Geometry check sheet. Reference: the model listing, model coordinates, mm. A direction names the side the tool comes from. Coordinates: 2 decimals unless noted, no trailing zeros. Write each loop counter-clockwise with the first axis right and the second up, starting at its lowest first coordinate (ties: lowest second). Pieces come first, ordered by that corner, then holes.
from build123d import *

# Parameters (mm, degrees)
SKETCH1_W              = 34.925
SKETCH1_H              = 31.75
PLATE_DEPTH            = 4
F_10_CLEARANCE_HOLE1_D = 5.1054
LOAD_CELL_CUTOUT_REACH = 26.919
FILLET1_R              = 3.175
CUT_EXTRUDE1_REACH     = 26.919
SKETCH5_R              = 2.6035
CHAMFER1_SIZE          = 0.508


with BuildPart() as part:
    # Sketch1 → Plate (new, symmetric)
    with BuildSketch(Plane(origin=(0, 0, 0), x_dir=(1, 0, 0), z_dir=(0, 1, 0))):
        Rectangle(SKETCH1_W, SKETCH1_H)
    extrude(amount=PLATE_DEPTH, both=True)

    # #10 Clearance Hole1 (through all)
    with Locations(Plane(origin=(0, 4, 0), x_dir=(1, 0, 0), z_dir=(0, 1, 0))):
        with Locations((-12.7, 11.1125), (12.7, 11.1125), (12.7, -11.1125), (-12.7, -11.1125)):
            Hole(F_10_CLEARANCE_HOLE1_D / 2)

    # Sketch4 → Load Cell Cutout (cut, up to next)
    with BuildSketch(Plane(origin=(0, 4, 0), x_dir=(1, 0, 0), z_dir=(0, 1, 0)), mode=Mode.PRIVATE) as load_cell_cutout_sk1:
        with BuildLine():
            Line((11.009869163, 6.927542495), (17.078427656, 5.008))
            Line((17.078427656, 5.008), (22.733, 5.008))
            Line((22.733, 5.008), (22.733, -5.008))
            Line((22.733, -5.008), (17.078427656, -5.008))
            Line((17.078427656, -5.008), (11.009869163, -6.927542495))
            ThreePointArc((11.009869163, -6.927542495), (-13.008, 0), (11.009869163, 6.927542495))
        make_face()
    load_cell_cutout_tool1 = extrude(load_cell_cutout_sk1.sketch, amount=-LOAD_CELL_CUTOUT_REACH, mode=Mode.PRIVATE) & part.part
    add(load_cell_cutout_tool1.solids().sort_by_distance((2.977457, 4, 0))[0], mode=Mode.SUBTRACT)

    # Fillet1
    fillet1_edges = [part.edges().sort_by_distance(p)[0] for p in [
        (11.009869163, 0, 6.927542495),
        (11.009869163, 0, -6.927542495),
    ]]
    fillet(fillet1_edges, radius=FILLET1_R)

    # Sketch5 → Cut-Extrude1 (cut, up to next)
    with BuildSketch(Plane(origin=(0, 4, 0), x_dir=(1, 0, 0), z_dir=(0, 1, 0)), mode=Mode.PRIVATE) as cut_extrude1_sk1:
        with Locations(Location((-12.7, 11.1125, 0), (0, 0, 270))):
            Circle(SKETCH5_R)
    cut_extrude1_tool1 = extrude(cut_extrude1_sk1.sketch, amount=-CUT_EXTRUDE1_REACH, mode=Mode.PRIVATE) & part.part
    # Sketch5 → Cut-Extrude1 (cut, up to next)
    with BuildSketch(Plane(origin=(0, 4, 0), x_dir=(1, 0, 0), z_dir=(0, 1, 0)), mode=Mode.PRIVATE) as cut_extrude1_sk2:
        with Locations(Location((12.7, 11.1125, 0), (0, 0, 270))):
            Circle(SKETCH5_R)
    cut_extrude1_tool2 = extrude(cut_extrude1_sk2.sketch, amount=-CUT_EXTRUDE1_REACH, mode=Mode.PRIVATE) & part.part
    # Sketch5 → Cut-Extrude1 (cut, up to next)
    with BuildSketch(Plane(origin=(0, 4, 0), x_dir=(1, 0, 0), z_dir=(0, 1, 0)), mode=Mode.PRIVATE) as cut_extrude1_sk3:
        with Locations(Location((-12.7, -11.1125, 0), (0, 0, 270))):
            Circle(SKETCH5_R)
    cut_extrude1_tool3 = extrude(cut_extrude1_sk3.sketch, amount=-CUT_EXTRUDE1_REACH, mode=Mode.PRIVATE) & part.part
    # Sketch5 → Cut-Extrude1 (cut, up to next)
    with BuildSketch(Plane(origin=(0, 4, 0), x_dir=(1, 0, 0), z_dir=(0, 1, 0)), mode=Mode.PRIVATE) as cut_extrude1_sk4:
        with Locations(Location((12.7, -11.1125, 0), (0, 0, 270))):
            Circle(SKETCH5_R)
    cut_extrude1_tool4 = extrude(cut_extrude1_sk4.sketch, amount=-CUT_EXTRUDE1_REACH, mode=Mode.PRIVATE) & part.part
    add(cut_extrude1_tool1.solids().sort_by_distance((-12.7, 4, -11.1125))[0], mode=Mode.SUBTRACT)
    add(cut_extrude1_tool2.solids().sort_by_distance((12.7, 4, -11.1125))[0], mode=Mode.SUBTRACT)
    add(cut_extrude1_tool3.solids().sort_by_distance((-12.7, 4, 11.1125))[0], mode=Mode.SUBTRACT)
    add(cut_extrude1_tool4.solids().sort_by_distance((12.7, 4, 11.1125))[0], mode=Mode.SUBTRACT)

    # Chamfer1
    # the kernel refuses this chamfer: 0.508 mm, written as the material it takes off along each edge
    with BuildSketch(Plane(origin=(13.009505309, -4, -9.625084967), x_dir=(-0.30158215810749167, 0, 0.9534401931485937), z_dir=(0.9534401931485937, 0, 0.30158215810749167))) as chamfer1_piece_1:
        Polygon((3.175 - CHAMFER1_SIZE, 0), (3.175, -CHAMFER1_SIZE), (3.175, 0), align=None)
    revolve(axis=Axis((13.009505309, -4, -9.625084967), (0, -1, 0)), revolution_arc=35.951449602, mode=Mode.SUBTRACT)
    with BuildSketch(Plane(origin=(18.324016186, -4, -4.614008558), x_dir=(0.30146813499365677, -0.02749587661058555, -0.9530797135354744), z_dir=(-0.9534401931485939, 0, -0.30158215810749184)), Plane(origin=(12.051981957, -4, 6.597912354), x_dir=(0.30146813499365605, -0.02749587661058387, 0.9530797135354745), z_dir=(0.9534401931485941, 0, -0.30158215810749117))) as chamfer1_piece_2:
        Polygon((CHAMFER1_SIZE * 0.999621916911, -CHAMFER1_SIZE * 0.0274958766106), (-CHAMFER1_SIZE * 0.0274958766106, -CHAMFER1_SIZE * 0.999621916911), (0, 0), align=None)
    extrude(amount=6.578319516, mode=Mode.SUBTRACT)
    with BuildSketch(Plane(origin=(17.4625, -4, -3.701585042), x_dir=(-0.9996219169112968, -0.027495876610585605, 0), z_dir=(0, 0, -1)), Plane(origin=(17.4625, -4, 17.181414958), x_dir=(-0.9996219169112968, -0.027495876610585605, 0), z_dir=(0, 0, -1))) as chamfer1_piece_3:
        Polygon((CHAMFER1_SIZE * 0.999621916911, CHAMFER1_SIZE * 0.0274958766106), (-CHAMFER1_SIZE * 0.0274958766106, CHAMFER1_SIZE * 0.999621916911), (0, 0), align=None)
    extrude(amount=13.479829916, mode=Mode.SUBTRACT)
    with BuildSketch(Plane(origin=(18.768914958, -4, -15.875), x_dir=(0, -0.027495876610585605, 0.9996219169112968), z_dir=(-1, 0, 0)), Plane(origin=(-18.768914958, -4, 15.875), x_dir=(0, -0.027495876610585605, -0.9996219169112968), z_dir=(1, 0, 0))) as chamfer1_piece_4:
        Polygon((CHAMFER1_SIZE * 0.999621916911, CHAMFER1_SIZE * 0.0274958766106), (-CHAMFER1_SIZE * 0.0274958766106, CHAMFER1_SIZE * 0.999621916911), (0, 0), align=None)
    extrude(amount=37.537829916, mode=Mode.SUBTRACT)
    with BuildSketch(Plane(origin=(-17.4625, -4, -17.181414958), x_dir=(0.9996219169112968, -0.027495876610585605, 0), z_dir=(0, 0, 1))) as chamfer1_piece_5:
        Polygon((CHAMFER1_SIZE * 0.999621916911, CHAMFER1_SIZE * 0.0274958766106), (-CHAMFER1_SIZE * 0.0274958766106, CHAMFER1_SIZE * 0.999621916911), (0, 0), align=None)
    extrude(amount=34.362829916, mode=Mode.SUBTRACT)
    with BuildSketch(Plane(origin=(13.009505309, -4, 9.625084967), x_dir=(-0.8038994814723275, 0, -0.5947651836553002), z_dir=(-0.5947651836553002, 0, 0.8038994814723275))) as chamfer1_piece_6:
        Polygon((3.175 - CHAMFER1_SIZE, 0), (3.175, -CHAMFER1_SIZE), (3.175, 0), align=None)
    revolve(axis=Axis((13.009505309, -4, 9.625084967), (0, -1, 0)), revolution_arc=35.951449602, mode=Mode.SUBTRACT)
    with BuildSketch(Plane(origin=(0, -4, 0), x_dir=(0.8038994814723273, 0, -0.5947651836553005), z_dir=(0.5947651836553005, 0, 0.8038994814723273))) as chamfer1_piece_7:
        Polygon((13.008 + CHAMFER1_SIZE, 0), (13.008, CHAMFER1_SIZE), (13.008, 0), align=None)
    revolve(axis=Axis((0, -4, 0), (0, 1, 0)), revolution_arc=287.00821123, mode=Mode.SUBTRACT)
    with BuildSketch(Plane(origin=(-12.7, -4, -11.1125), x_dir=(0, 0, 1), z_dir=(-1, 0, 0))) as chamfer1_piece_8:
        Polygon((2.6035 + CHAMFER1_SIZE, 0), (2.6035, CHAMFER1_SIZE), (2.6035, 0), align=None)
    revolve(axis=Axis((-12.7, -4, -11.1125), (0, 1, 0)), mode=Mode.SUBTRACT)
    with BuildSketch(Plane(origin=(12.7, -4, -11.1125), x_dir=(0, 0, 1), z_dir=(-1, 0, 0))) as chamfer1_piece_9:
        Polygon((2.6035 + CHAMFER1_SIZE, 0), (2.6035, CHAMFER1_SIZE), (2.6035, 0), align=None)
    revolve(axis=Axis((12.7, -4, -11.1125), (0, 1, 0)), mode=Mode.SUBTRACT)
    with BuildSketch(Plane(origin=(-12.7, -4, 11.1125), x_dir=(0, 0, 1), z_dir=(-1, 0, 0))) as chamfer1_piece_10:
        Polygon((2.6035 + CHAMFER1_SIZE, 0), (2.6035, CHAMFER1_SIZE), (2.6035, 0), align=None)
    revolve(axis=Axis((-12.7, -4, 11.1125), (0, 1, 0)), mode=Mode.SUBTRACT)
    with BuildSketch(Plane(origin=(12.7, -4, 11.1125), x_dir=(0, 0, 1), z_dir=(-1, 0, 0))) as chamfer1_piece_11:
        Polygon((2.6035 + CHAMFER1_SIZE, 0), (2.6035, CHAMFER1_SIZE), (2.6035, 0), align=None)
    revolve(axis=Axis((12.7, -4, 11.1125), (0, 1, 0)), mode=Mode.SUBTRACT)


solid = part.part
1. Draft check along Z on faces 1 (the cylindrical face through (-10.12, 0.31, 10.77)), 2 (the flat face through (0, 0, -15.875)), 3 (the flat face through (17.462, 0, 11)). Enter one of: released by +Z, released by -Z, zero draft, split by the parting line, or undercut.
Computed values:
face 1: undercut
face 2: released by -Z
face 3: zero draft
2. Sectioned sample at C-C, the plane z = 0. Record the boundary of the cut face in (x, y).
Computed values:
outline: (-17.46, -3.49) - (-16.95, -4) - (-13.52, -4) - (-13.01, -3.49) - (-13.01, 4) - (-17.46, 4) - close
3. Sectioned sample at B-B, the plane y = -2. Give the number of separate pieces and of enclosed holes in the cut face, and give its area (3 significant figures).
Computed values:
separate pieces: 1
enclosed holes: 4
area: 434 mm2
4. Sectioned sample at D-D, the plane x = 12.7. Record the boundary of the cut face in (y, z) (3 decimals), and give its area (3 significant figures).
Computed values:
outline: (-4, -15.367) - (-3.492, -15.875) - (4, -15.875) - (4, -13.716) - (-3.492, -13.716) - (-4, -14.224) - close; (-4, -8.001) - (-3.492, -8.509) - (4, -8.509) - (4, -6.393) - (-3.492, -6.393) - (-4, -6.926) - close; (-4, 6.926) - (-3.492, 6.393) - (4, 6.393) - (4, 8.509) - (-3.492, 8.509) - (-4, 8.001) - close; (-4, 14.224) - (-3.492, 13.716) - (4, 13.716) - (4, 15.875) - (-3.492, 15.875) - (-4, 15.367) - close
area: 67.4 mm2
5. Sectioned sample at A-A, the plane x = 0. Record the boundary of the cut face in (y, z) (3 decimals).
Computed values:
outline: (-4, -15.367) - (-3.492, -15.875) - (4, -15.875) - (4, -13.008) - (-3.492, -13.008) - (-4, -13.516) - close; (-4, 13.516) - (-3.492, 13.008) - (4, 13.008) - (4, 15.875) - (-3.492, 15.875) - (-4, 15.367) - close
6. Gauge pin test, flat end, axial feed: pin 1 Ø6 at (x, z) = (12.7, -11.11) entering from -Y. Record the tip position at first contact, or that the pin passes through.
Computed values:
pin 1: stops at y = -3.89
7. Thickness scan on line 1 along Z through (x, y) = (14.5, 1.25) (3 decimals); line 2 along Z through (x, y) = (15, -2) (3 decimals); line 3 along Z through (x, y) = (0, 2.25) (3 decimals). Record the ranges inside material, lowest first.
Computed values:
line 1: z = -15.875 to -12.994, -9.231 to -5.824, 5.824 to 9.231, 12.994 to 15.875
line 2: z = -15.875 to -12.332, -9.893 to -5.665, 5.665 to 9.893, 12.332 to 15.875
line 3: z = -15.875 to -13.008, 13.008 to 15.875
8. Access from +Z, -Z, +X, -X, +Y, -Y to the whole of each face (thin tool, end or side, straight path). Record for faces 4 (the flat face through (14.6, 0.31, 5.79)), 5 (the flat face through (0, 0, 15.875)), 6 (the flat face through (14.74, -3.75, 6.02)).
Computed values:
face 4: +Y, -Y
face 5: +Z, +X, -X, +Y, -Y
face 6: -Y
